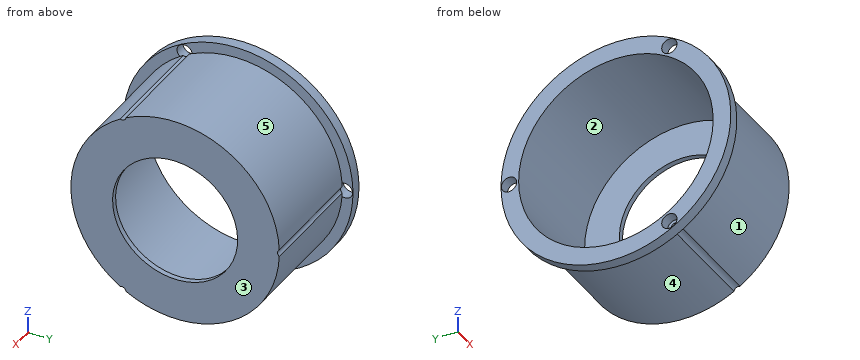
from build123d import *

# Parameters (mm, degrees)
AXIAL_HOLES_DEPTH      = 192.606080279
AXIAL_HOLES_DEPTH_BACK = 192.606080279
SKETCH2_R              = 1.65
CUT_EXTRUDE2_START     = 135.7
SKETCH3_R              = 2.85
CUT_EXTRUDE2_DEPTH     = 4


with BuildPart() as part:
    # Axial profile (mm) → Full revolution (revolve)
    with BuildSketch(Plane.XY, mode=Mode.PRIVATE) as full_revolution_sk:
        Polygon((135.7, 36.4), (179.7, 36.4), (179.7, 23.4), (181.7, 23.4), (181.7, 39), (139.7, 39), (139.7, 43), (135.7, 43), align=None)
    revolve(full_revolution_sk.sketch.rotate(Axis((-110, 0, 0), (1, 0, 0)), 90), axis=Axis((-110, 0, 0), (1, 0, 0)))

    # Sketch2 → Axial holes (cut, two sides: drawn at the far end of the back side and taken through both)
    with BuildSketch(Plane(origin=(0, 0, 0), x_dir=(0, 0, -1), z_dir=(1, 0, 0)).offset(-AXIAL_HOLES_DEPTH_BACK)):
        with Locations(Location((0, 40, 0), (0, 0, 218.251159994))):
            Circle(SKETCH2_R)
        with Locations(Location((-34.641016151, -20, 0), (0, 0, 81.748840006))):
            Circle(SKETCH2_R)
        with Locations(Location((34.641016151, -20, 0), (0, 0, 201.748840006))):
            Circle(SKETCH2_R)
    extrude(amount=AXIAL_HOLES_DEPTH + AXIAL_HOLES_DEPTH_BACK, mode=Mode.SUBTRACT)

    # Sketch3 → Cut-Extrude2 (cut)
    with BuildSketch(Plane(origin=(0, 0, 0), x_dir=(0, 0, -1), z_dir=(1, 0, 0)).offset(CUT_EXTRUDE2_START)):
        with Locations(Location((0, 40, 0), (0, 0, 202.464828441))):
            Circle(SKETCH3_R)
        with Locations(Location((-34.641016151, -20, 0), (0, 0, 97.535171559))):
            Circle(SKETCH3_R)
        with Locations(Location((34.641016151, -20, 0), (0, 0, 217.535171559))):
            Circle(SKETCH3_R)
    extrude(amount=CUT_EXTRUDE2_DEPTH, mode=Mode.SUBTRACT)


solid = part.part
Can you work these out from the model? Positions are in its coordinate system, mm. Face numbers are marked on the shaded views. A direction names the side the tool comes from. Coordinates: 2 decimals unless noted, no trailing zeros. Loops run counter-clockwise (first coordinate to the right, second up) from the corner with the lowest first, then second, coordinate; pieces in that order, holes last. Notation, with made-up numbers: (-17.75, 28) - (7.25, 28) arc R33 ccw to (7.25, 58) - close; hole circle Ø5 at (69, 19.25). An arc over 180 degrees is marked (long way). Put each result on its own line as item: value. Start each with the question number.
Item 1: Suppose I cut it at B-B (y = 0). Please give me the cut outline in (x, z), and give its area (3 significant figures).
Item 2: If I drill on line 1 along Y through (x, z) = (166, 0); line 2 along Z through (x, y) = (137.65, -20); line 3 along X through (y, z) = (23, -7), over which ranges is the centre line in solid material (lowest first)?
Item 3: Suppose I cut it at D-D (z = 9). Please give me the cut outline in (x, y).
Item 4: For pin 1 (5 mm diameter, centred on y = -20, z = 34.64, fed in from -X); pin 2 (12 mm diameter, centred on x = 165.5, z = 24.5, fed in from +Y); pin 3 (1.5 mm diameter, centred on x = 170, z = -14.5, fed in from +Y), each with a flat end and sliding along its axis, tell me the tip position at first contact or that it passes through.
Item 5: Suppose I cut it at C-C (x = 161). Please give me the cut outline in (y, z).
Item 6: Suppose I cut it at A-A (z = 0). Please give me the cut outline in (x, y).
Item 7: Which directions (+Z, -Z, +X, -X, +Y, -Y) give clear straight access to the entire face, cutting with the end or side of a thin tool? Please do the marked faces 1, 2, 3, 4 and 5.
Here are the results:
1. outline: (135.7, -43) - (139.7, -43) - (139.7, -39) - (181.7, -39) - (181.7, -23.4) - (179.7, -23.4) - (179.7, -36.4) - (135.7, -36.4) - close; (135.7, 36.4) - (179.7, 36.4) - (179.7, 23.4) - (181.7, 23.4) - (181.7, 39) - (139.7, 39) - (139.7, 43) - (135.7, 43) - close
1. area: 323 mm²
2. line 1: -39 to -36.4, 36.4 to 38.35
2. line 2: -38.07 to -37.49, -31.79 to -30.41, 30.41 to 31.79, 37.49 to 38.07
2. line 3: 179.7 to 181.7
3. outline: (135.7, -42.05) - (139.7, -42.05) - (139.7, -37.95) - (181.7, -37.95) - (181.7, -21.6) - (179.7, -21.6) - (179.7, -35.27) - (135.7, -35.27) - close; (135.7, 35.27) - (179.7, 35.27) - (179.7, 21.6) - (181.7, 21.6) - (181.7, 37.95) - (139.7, 37.95) - (139.7, 42.05) - (135.7, 42.05) - close
4. pin 1: x = 139.7
4. pin 2: y = 34.33
4. pin 3: y = 36.5
5. outline: (-20.61, -33.11) arc R1.65 cw to (-18.37, -34.4) arc R39 ccw to (38.98, -1.3) arc R1.65 cw to (38.98, 1.3) arc R39 ccw to (-18.37, 34.4) arc R1.65 cw to (-20.61, 33.11) arc R39 ccw to start; hole circle Ø72.8 at (0, 0)
6. outline: (135.7, -43) - (139.7, -43) - (139.7, -39) - (181.7, -39) - (181.7, -23.4) - (179.7, -23.4) - (179.7, -36.4) - (135.7, -36.4) - close; (135.7, 36.4) - (179.7, 36.4) - (179.7, 23.4) - (181.7, 23.4) - (181.7, 38.35) - (139.7, 38.35) - (139.7, 37.15) - (135.7, 37.15) - close; (135.7, 42.85) - (139.7, 42.85) - (139.7, 43) - (135.7, 43) - close
7. face 1: +X, -Y
7. face 2: -X
7. face 3: +Z, -Z, +X, +Y, -Y
7. face 4: -Z, +X
7. face 5: +Z, +X
